Source: three-view drawing plus pictorial views. Frame: mm from the lowest corner of the part. A direction names the side the tool comes from. Give positions to 0.01 mm unless a question says otherwise; leave off trailing zeros. Loops run counter-clockwise (first coordinate to the right, second up) from the corner with the lowest first, then second, coordinate; pieces in that order, holes last. Notation, with made-up numbers: (-3, 48) -> (5, 48) arc R26 ccw to (5, 66) -> close; hole circle Ø5 at (3.25, 24). An arc over 180 degrees is marked (long way). Answer as a JSON object with one key per item and string values. Group by question number.
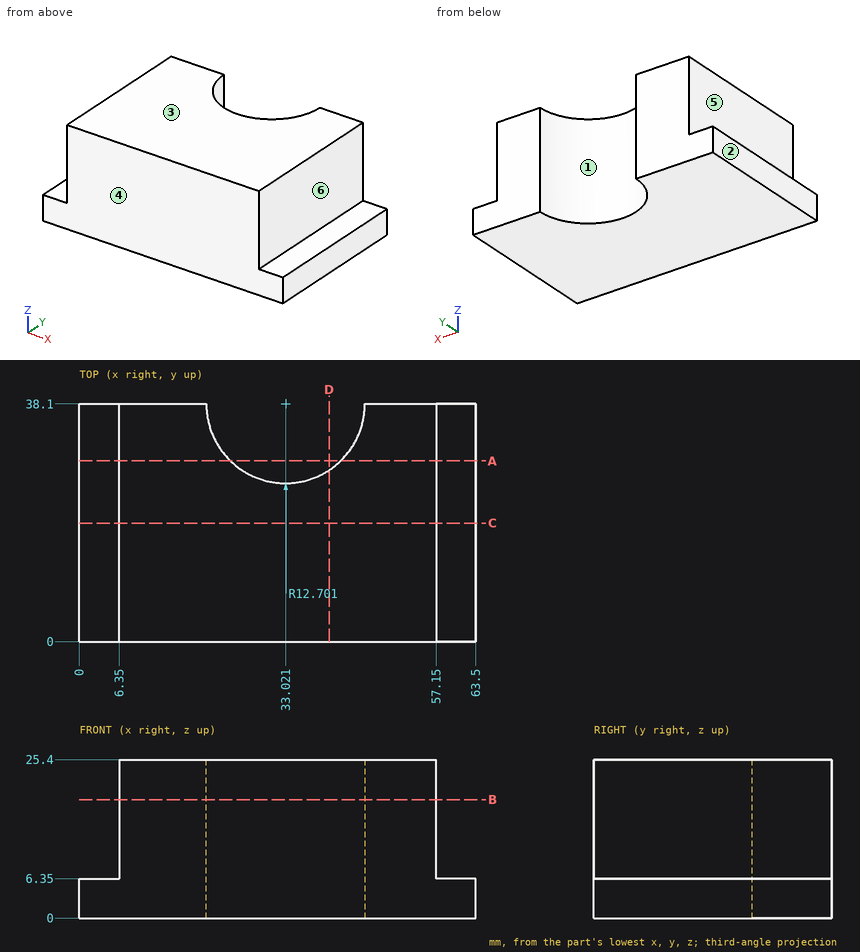
Q1. Section D-D on x = 40. Return the cut outline in (y, z), then the cut area to 3 significant figures.
Q2. Set-up query: the marked faces 4, 5 and 6. Return all of +Z, -Z, +X, -X, +Y, -Y with unobstructed straight access to the full face (end or side cutting, diameter ignored); none if empty.
Q3. Pull-direction query (X, two-part tool) for the marked faces 1, 2 and 3; classes: +X half, -X half, draft (parallel to the pull), parting line (faces both ways), or undercut.
Q4. Section B-B on z = 19. Return the cut outline in (x, y), then the cut area to 3 significant figures.
Q5. Section A-A on y = 29. Return the cut outline in (x, z), then the cut area to 3 significant figures.
Q6. Ray query, probe 1 along X at (y, z) = (14, 15.25); probe 2 along Z at (x, y) = (57.5, 8); probe 3 along Y at (x, z) = (22, 16.75) (1 decimal). Return the intervals inside material, ascending.
Q7. Pin query (flat end, axial travel): pin 1 Ø1.9 at (x, y) = (60.5, 22) entering from +Z; pin 2 Ø1 at (y, z) = (12, 18) entering from +X; pin 3 Ø2 at (y, z) = (19, 8) entering from -X. Return the tip coordinate at first contact, or that it passes through.
Q8. Section C-C on y = 19. Return the cut outline in (x, z).
Numbers:
{
 "1": {"outline": "(0, 0) -> (27.49, 0) -> (27.49, 25.4) -> (0, 25.4) -> close", "area": "698 mm²"},
 "2": {"face 4": "+Z, -Z, +X, -X, -Y", "face 5": "+Z, -X, +Y, -Y", "face 6": "+Z, +X, +Y, -Y"},
 "3": {"face 1": "undercut", "face 2": "-X half", "face 3": "draft"},
 "4": {"outline": "(6.35, 0) -> (57.15, 0) -> (57.15, 38.1) -> (45.72, 38.1) arc R12.7 cw to (20.32, 38.1) -> (6.35, 38.1) -> close", "area": "1,680 mm²"},
 "5": {"outline": "(0, 0) -> (24.16, 0) -> (24.16, 25.4) -> (6.35, 25.4) -> (6.35, 6.35) -> (0, 6.35) -> close; (41.88, 0) -> (63.5, 0) -> (63.5, 6.35) -> (57.15, 6.35) -> (57.15, 25.4) -> (41.88, 25.4) -> close", "area": "921 mm²"},
 "6": {"probe 1": "x = 6.35 to 57.15", "probe 2": "z = 0 to 6.35", "probe 3": "y = 0 to 31.8"},
 "7": {"pin 1": "stops at z = 6.35", "pin 2": "stops at x = 57.15", "pin 3": "stops at x = 6.35"},
 "8": {"outline": "(0, 0) -> (63.5, 0) -> (63.5, 6.35) -> (57.15, 6.35) -> (57.15, 25.4) -> (6.35, 25.4) -> (6.35, 6.35) -> (0, 6.35) -> close"}
}
